from build123d import *

# Parameters (mm, degrees)
BOSS_EXTRUDE1_DEPTH   = 11.5
BOSS_EXTRUDE1_2_DEPTH = 11.5
BOSS_EXTRUDE1_3_DEPTH = 11.5
SKETCH2_W             = 34.3
SKETCH2_H             = 10.7
BOSS_EXTRUDE2_DEPTH   = 5.1
FILLET1_R             = 1


with BuildPart() as part:
    # Sketch1 → Boss-Extrude1 (new body)
    with BuildSketch(Plane(origin=(0, 0, 0), x_dir=(1, 0, 0), z_dir=(0, 1, 0))):
        with BuildLine():
            ThreePointArc((-11.848101114, 5.35), (-13, 0), (-11.848101114, -5.35))
            Line((-11.848101114, -5.35), (-17.15, -5.35))
            Line((-17.15, -5.35), (-17.15, 5.35))
            Line((-17.15, 5.35), (-11.848101114, 5.35))
        make_face()
    extrude(amount=BOSS_EXTRUDE1_DEPTH)



with BuildPart() as body_2:
    # Sketch1 → Boss-Extrude1 2 (new body)
    with BuildSketch(Plane(origin=(0, 0, 0), x_dir=(1, 0, 0), z_dir=(0, 1, 0))):
        with BuildLine():
            Line((0.733143915, 5.35), (-0.733143915, 5.35))
            ThreePointArc((-0.733143915, 5.35), (-5.4, 0), (-0.733143915, -5.35))
            Line((-0.733143915, -5.35), (0.733143915, -5.35))
            ThreePointArc((0.733143915, -5.35), (4.069335151, -3.549719909), (5.4, 0))
            ThreePointArc((5.4, 0), (4.069335151, 3.549719909), (0.733143915, 5.35))
        make_face()
    extrude(amount=BOSS_EXTRUDE1_2_DEPTH)


with BuildPart() as body_3:
    # Sketch1 → Boss-Extrude1 3 (new body)
    with BuildSketch(Plane(origin=(0, 0, 0), x_dir=(1, 0, 0), z_dir=(0, 1, 0))):
        with BuildLine():
            ThreePointArc((11.848101114, -5.35), (13, 0), (11.848101114, 5.35))
            Line((11.848101114, 5.35), (17.15, 5.35))
            Line((17.15, 5.35), (17.15, -5.35))
            Line((17.15, -5.35), (11.848101114, -5.35))
        make_face()
    extrude(amount=BOSS_EXTRUDE1_3_DEPTH)


with BuildPart() as part_1:
    add(part.part)

    add(body_2.part)  # Boss-Extrude2 merges body 2

    add(body_3.part)  # Boss-Extrude2 merges body 3
    # Sketch2 → Boss-Extrude2 (add)
    with BuildSketch(Plane.XZ):
        Rectangle(SKETCH2_W, SKETCH2_H)
    extrude(amount=BOSS_EXTRUDE2_DEPTH)

    # Fillet1
    fillet1_edges = [part_1.edges().sort_by_distance(p)[0] for p in [
        (-6.290622514, 0, -5.35),
        (6.290622514, 0, -5.35),
        (-6.290622514, 0, 5.35),
        (6.290622514, 0, 5.35),
        (11.848101114, 5.75, -5.35),
        (11.848101114, 5.75, 5.35),
        (-11.848101114, 5.75, 5.35),
        (-11.848101114, 5.75, -5.35),
    ]]
    fillet(fillet1_edges, radius=FILLET1_R)


solid = part_1.part
Design review of the part built by this model. Coordinates are the model's own, in mm. A direction names the side the tool comes from. Coordinates: 2 decimals unless noted, no trailing zeros. Write each loop counter-clockwise with the first axis right and the second up, starting at its lowest first coordinate (ties: lowest second). Pieces come first, ordered by that corner, then holes. Notation, with made-up numbers: (18.5, 13.5) - (32.5, 13.5) arc R17 ccw to (32.5, 31.5) - close; hole circle Ø1 at (69, -11.75). An arc over 180 degrees is marked (long way). Use one line per item in the form item = value.
Q1. Consider section B-B (z = -1.75). Write out the cut boundary in (x, y).
Taken from the geometry:
outline = (-17.15, -5.1) - (17.15, -5.1) - (17.15, 11.5) - (12.88, 11.5) - (12.88, 0) - (5.11, 0) - (5.11, 11.5) - (-5.11, 11.5) - (-5.11, 0) - (-12.88, 0) - (-12.88, 11.5) - (-17.15, 11.5) - close
Q2. Consider section C-C (x = -4). Write out the cut boundary in (y, z).
Taken from the geometry:
outline = (-5.1, -5.35) - (-1, -5.35) arc R1 ccw to (0, -4.35) - (0, -3.63) - (11.5, -3.63) - (11.5, 3.63) - (0, 3.63) - (0, 4.35) arc R1 ccw to (-1, 5.35) - (-5.1, 5.35) - close
Q3. Machinability: for faces 4 (the cylindrical face through (7.108, -0.301, -5.065)), 5 (the cylindrical face through (-6.932, -0.285, 5.049)), 6 (the cylindrical face through (12.49, 5.34, 4.93)), which of the approach directions +Z, -Z, +X, -X, +Y, -Y give a long, thin tool a straight path to every point of the face, cutting with its end or side? Answer none if there is none.
Taken from the geometry:
face_4 = -Z, +Y
face_5 = +Z, +Y
face_6 = +Y
Q4. Insertion check: pin 1 Ø2 at (x, z) = (6.5, 1) entering from +Y. The pin has a flat end and moves straight along its axis. Give the tip position at first contact, or say it passes through.
Taken from the geometry:
pin_1 = 0
Q5. The part is to be moulded in two halves that separate along X. For faces 1 (the flat face through (0, 11.5, 0)), 2 (the flat face through (-17.15, 3, 0)), 3 (the cylindrical face through (-6.932, -0.301, -5.065)), say which applies: +X half, -X half, draft (parallel to the pull), parting line (faces both ways), or undercut.
Taken from the geometry:
face_1 = draft
face_2 = -X half
face_3 = undercut
Q6. For probe 1 along X at (y, z) = (7, -1.75); probe 2 along X at (y, z) = (9, -0.5); probe 3 along Y at (x, z) = (10.5, -2.5), list the stretches that pass through material, from the lowest coordinate up.
Taken from the geometry:
probe_1 = -17.15 to -12.88, -5.11 to 5.11, 12.88 to 17.15
probe_2 = -17.15 to -12.99, -5.38 to 5.38, 12.99 to 17.15
probe_3 = -5.1 to 0
Q7. Consider section D-D (z = 0.75). Write out the cut boundary in (x, y).
Taken from the geometry:
outline = (-17.15, -5.1) - (17.15, -5.1) - (17.15, 11.5) - (12.98, 11.5) - (12.98, 0) - (5.35, 0) - (5.35, 11.5) - (-5.35, 11.5) - (-5.35, 0) - (-12.98, 0) - (-12.98, 11.5) - (-17.15, 11.5) - close
Q8. Consider section A-A (y = 1.5). Write out the cut boundary in (x, z), plus the area to 3 significant figures.
Taken from the geometry:
outline = (-17.15, -5.35) - (-13.31, -5.35) arc R1 ccw to (-12.36, -4.04) arc R13 cw to (-12.36, 4.04) arc R1 ccw to (-13.31, 5.35) - (-17.15, 5.35) - close; (-0.73, -5.35) - (0.73, -5.35) arc R5.4 ccw to (0.73, 5.35) - (-0.73, 5.35) arc R5.4 ccw to start; (12.36, -4.04) arc R1 ccw to (13.31, -5.35) - (17.15, -5.35) - (17.15, 5.35) - (13.31, 5.35) arc R1 ccw to (12.36, 4.04) arc R13 cw to start
area = 187 mm^2
